The listing builds one solid part. Answer for the finished solid, in the listing's coordinates (mm). A direction names the side the tool comes from. Coordinates: 2 decimals unless noted, no trailing zeros. Write each loop counter-clockwise with the first axis right and the second up, starting at its lowest first coordinate (ties: lowest second). Pieces come first, ordered by that corner, then holes. Notation, with made-up numbers: M 32.5,81.5 L 73.5,81.5 A11 cw 73.5,87.5 Z; hole C 38,15 d8. An arc over 180 degrees is marked long. Answer as CSV lines item,"result".
```python
from build123d import *

# Parameters (mm, degrees)
ESTRUSIONE_ESTRUSIONE1_DEPTH = 60
SCHIZZO2_R                   = 53
TAGLIO_ESTRUSIONE1_DEPTH     = 60
SCHIZZO3_R                   = 60
TAGLIO_ESTRUSIONE2_DEPTH     = 21


with BuildPart() as part:
    # Schizzo1 → Estrusione-Estrusione1 (new body)
    with BuildSketch(Plane.XY):
        Polygon((-65, 26), (0, 26), (0, 16), (-15, 16), (-15, 0), (51.592663953, 0), (0, 31), (-65, 31), align=None)
    extrude(amount=ESTRUSIONE_ESTRUSIONE1_DEPTH)

    # Schizzo2 → Taglio-Estrusione1 (cut)
    with BuildSketch(Plane(origin=(0, 31, 0), x_dir=(1, 0, 0), z_dir=(0, 1, 0))):
        with Locations((-68, -30)):
            Circle(SCHIZZO2_R)
    extrude(amount=-TAGLIO_ESTRUSIONE1_DEPTH, mode=Mode.SUBTRACT)

    # Schizzo3 → Taglio-Estrusione2 (cut)
    with BuildSketch(Plane.XZ):
        with Locations((-68, 30)):
            Circle(SCHIZZO3_R)
    extrude(amount=-TAGLIO_ESTRUSIONE2_DEPTH, mode=Mode.SUBTRACT)


solid = part.part
```
Q1. The mould has two halves that part along Y. Classify faces 4 (the flat face through (18, 0, 30)), 5 (the flat face through (-10, 26, 30)), 6 (the flat face through (-6, 16, 30)), 7 (the cylindrical face through (-15, 29, 30)): pulls with the +Y half, pulls with the -Y half, needs draft (parallel to the pull), parting line crosses it, or undercut.
Output:
face 4,"pulls with the -Y half"
face 5,"undercut"
face 6,"undercut"
face 7,"needs draft"
Q2. For faces 1 (the flat face through (0, 21, 30)), 2 (the cylindrical face through (-8, 8, 30)), 3 (the flat face through (-15, 8, 1)), determine the directions among +Z, -Z, +X, -X, +Y, -Y from which every point of the face is accessible in a straight line to the end or side of a thin tool.
Output:
face 1,"+Z, -Z, -X"
face 2,"-X, -Y"
face 3,"+Z, -Z, -X, -Y"
Q3. Find section A-A (y = 14). Give the vertices of the cut face in (x, z), and give its area (3 significant figures).
Output:
outline,"M -15,0 L 28.29,0 L 28.29,60 L -15,60 L -15,58.12 A60 cw -15,1.88 Z"
area,"2,330 mm2"
Q4. Straight lines are drawn through the part: line 1 (Y direction, x = -1, z = 56); line 2 (Y direction, x = -12, z = 34); line 3 (X direction, y = 6, z = 16.5). For each, find the intervals that lie inside material, in ascending order.
Output:
line 1,"0 to 16, 26 to 31"
line 2,"26 to 31"
line 3,"-9.54 to 41.61"
Q5. Flat-ended cylindrical pins translate along their axes: pin 1 Ø2 at (y, z) = (22, 18) entering from +X; pin 2 Ø3 at (y, z) = (25.5, 40.5) entering from +X; pin 3 Ø12 at (y, z) = (26.5, 28.5) entering from +X. Find the tip coordinate at first contact, or state that the pin passes through.
Output:
pin 1,"x = 16.64"
pin 2,"x = 11.65"
pin 3,"x = 17.47"
Q6. Find section D-D (y = 8). Give the vertices of the cut face in (x, z).
Output:
outline,"M -15,0 L 38.28,0 L 38.28,60 L -15,60 L -15,58.12 A60 cw -15,1.88 Z"
Q7. Find section B-B (z = 51). Give the vertices of the cut face in (x, y), and give its area (3 significant figures).
Output:
outline,"M -19.34,26 L 0,26 L 0,16 L -11.8,16 L -11.8,0 L 51.59,0 L 0,31 L -19.34,31 Z"
area,"1,090 mm2"
Q8. Find section C-C (x = 14.5). Give the vertices of the cut face in (y, z), and give its area (3 significant figures).
Output:
outline,"M 0,0 L 22.29,0 L 22.29,60 L 0,60 Z"
area,"1,340 mm2"
